Autodesk Inventor part; units mm, degrees
ref_plane "Work Plane1" through (0, 3.2, 0) normal (0, 1, 0) x (1, 0, 0)
ref_plane "YZ Plane" through (0, 0, 0) normal (1, 0, 0) x (0, 1, 0)
ref_plane "XZ Plane" through (0, 0, 0) normal (0, 1, 0) x (-1, 0, 0)
sketch "Sketch1" plane through (0, 0, 0) normal (0, 1, 0) x (-1, 0, 0)
  line L0 (0, 0) -> (0, -10.2)
  line L1 (0, -10.2) -> (-8.8, -10.2)
  line L2 (-8.8, -10.2) -> (-9.5, -9.5)
  line L3 (-9.5, -9.5) -> (-19.8, -9.5)
  line L4 (-19.8, -9.5) -> (-19.8, 0)
  line L5 (-19.8, 0) -> (0, 0)
  dimension "d0" = 10.2
  dimension "d1" = 9.5
  dimension "ss5glfLength" = 19.8
  dimension "d4" = 8.8
  dimension "d5" = 135
extrude "Extrusion1" add sketch "Sketch1" along normal blind 6.4
sketch "Sketch2" plane through (0, 0, 0) normal (0, 0, 1) x (1, 0, 0)
  line L0 (1.6, 4.8) -> (2.06, 4.8)
  line L1 (2.06, 4.8) -> (2.06, 1.6)
  line L2 (2.06, 1.6) -> (1.6, 1.6)
  line L3 (1.6, 1.6) -> (1.6, 4.8)
  line L4 (10.4, 4.8) -> (10.86, 4.8)
  line L5 (10.86, 4.8) -> (10.86, 1.6)
  line L6 (10.86, 1.6) -> (10.4, 1.6)
  line L7 (10.4, 1.6) -> (10.4, 4.8)
  line L8 (0, 0) -> (0, 6.4)
  line L9 (19.8, 0) -> (0, 0)
  dimension "d8" = 0.46
  dimension "pinWidth" = 3.2
  dimension "d10" = 1.6
  dimension "d11" = 8.8
  dimension "d12" = 1.6
extrude "Extrusion2" add sketch "Sketch2" along normal blind 3.9
ref_plane "Work Plane1" through (0, 3.2, 0) normal (0, 1, 0) x (1, 0, 0)
sketch "Sketch3" plane through (0, 3.2, 0) normal (0, 1, 0) x (1, 0, 0)
  line L0 (8.8, 10.2) -> (0, 10.2)
  line L1 (3.1, 10.2) -> (3.1, 11.1084)
  line L2 (3.1, 11.1084) -> (18.9478, 12.4949)
  line L3 (18.9478, 12.4949) -> (18.9391, 12.5945)
  line L4 (18.9391, 12.5945) -> (3, 11.2)
  line L5 (3, 11.2) -> (3, 10.2)
  line L6 (0, 10.2) -> (0, 0)
  dimension "d15" = 16
  dimension "d16" = 1
  dimension "d17" = 0.1
  dimension "d18" = 0.1
  dimension "d19" = 95
  dimension "d20" = 3
extrude "Extrusion3" add sketch "Sketch3" along normal mid plane 3.6
equation "\"d12\" = -0.5 * pinWidth + 0.5 * width"
properties part number "SS-5GL-F"
Build history of the part. All positions in model axes, mm. A direction names the side the tool comes from. Round coordinates to 2 decimals unless told otherwise and drop trailing zeros. Write each loop counter-clockwise with the first axis right and the second up, starting at its lowest first coordinate (ties: lowest second). Pieces come first, ordered by that corner, then holes. Notation, with made-up numbers: M 44,-27.75 L 54,-27.75 A25 cw 54,3.25 Z; hole C 23.5,17 d2. An arc over 180 degrees is marked long. Answer as a JSON object with one key per item and string values. Group by question number.
(1) Cut at C-C (x = 2.5). Give the cut face in (y, z).
(2) Cut at B-B (y = 3.25). Give the cut face in (x, z), and give its area (3 significant figures).
(3) Cut at A-A (x = 15). Give the cut face in (y, z), and give its area (3 significant figures).
(4) Cut at D-D (z = -10.5). Give the cut face in (x, y).
(5) Mould opens along X. For faces 1 (the flat face through (1.6, 3, 2)), 2 (the flat face through (4, 3, -10.2)), 3 (the flat face through (10, 3, 0)) say: pulls with the +X half, pulls with the -X half, needs draft (parallel to the pull), parting line crosses it, or undercut.
(6) Flat gauge pins, fed straight in: pin 1 (3 mm diameter, centred on x = 13, y = 5.5, fed in from -Z); pin 2 (1.6 mm diameter, centred on y = 3.5, z = 1.5, fed in from +X); pin 3 (2.5 mm diameter, centred on x = 12.5, z = -11.5, fed in from +Y). Where does each tip first touch, or does it go through?
(7) Drill centre lines: L1, parallel to X at y = 3.5, z = 0.75; L2, parallel to Z at x = 10, y = 0.5; L3, parallel to Z at x = 4, y = 0.5. Where is each one in solid material? Low to high.
(8) Which spindle directions (+Z, -Z, +X, -X, +Y, -Y) get a long thin tool onto all of the face, cutting with end or side? Do faces 4 (the flat face through (10, 0, -5)), 5 (the flat face through (10.4, 3, 2)), 6 (the flat face through (10.86, 3, 2)), 7 (the flat face through (15, 3, -9.5)), 8 (the flat face through (19.8, 3, -5)). Say none if no direction does.
Responses:
{
 "1": {"outline": "M 0,-10.2 L 6.4,-10.2 L 6.4,0 L 0,0 Z"},
 "2": {"outline": "M 0,-10.2 L 3,-10.2 L 3,-11.2 L 18.94,-12.59 L 18.95,-12.49 L 3.1,-11.11 L 3.1,-10.2 L 8.8,-10.2 L 9.5,-9.5 L 19.8,-9.5 L 19.8,0 L 10.86,0 L 10.86,3.9 L 10.4,3.9 L 10.4,0 L 2.06,0 L 2.06,3.9 L 1.6,3.9 L 1.6,0 L 0,0 Z", "area": "200 mm2"},
 "3": {"outline": "M 0,-9.5 L 6.4,-9.5 L 6.4,0 L 0,0 Z; M 1.4,-12.25 L 5,-12.25 L 5,-12.15 L 1.4,-12.15 Z", "area": "61.2 mm2"},
 "4": {"outline": "M 3,1.4 L 3.1,1.4 L 3.1,5 L 3,5 Z"},
 "5": {"face 1": "pulls with the -X half", "face 2": "needs draft", "face 3": "undercut"},
 "6": {"pin 1": "stops at z = -12.2", "pin 2": "stops at x = 10.86", "pin 3": "stops at y = 5"},
 "7": {"L1": "x = 1.6 to 2.06, 10.4 to 10.86", "L2": "z = -9.5 to 0", "L3": "z = -10.2 to 0"},
 "8": {"face 4": "+Z, -Z, +X, -X, -Y", "face 5": "+Z, +Y, -Y", "face 6": "+Z, +X, +Y, -Y", "face 7": "+X, +Y, -Y", "face 8": "+Z, -Z, +X, +Y, -Y"}
}
